```python
from build123d import *

# Parameters (mm, degrees)
SKETCH_2_R          = 6.05
SKETCH_2_R_2        = 1.6
EXTRUDE_1_DEPTH     = 3
SKETCH_2_3_R        = 1.6
EXTRUDE_2_DEPTH     = 8
SKETCH_3_R          = 1.65
EXTRUDE_4_DEPTH     = 3
SKETCH_5_R          = 3
CUT_EXTRUDE_1_DEPTH = 3.5
SKETCH_6_W          = 55.305281636
SKETCH_6_H          = 51.082077229
CUT_EXTRUDE_2_DEPTH = 82.174934555
FILLET_10_R         = 6
FILLET_11_R         = 5


with BuildPart() as part:
    # ｽｹｯﾁ2 → ﾎﾞｽ - 押し出し1 (new body)
    with BuildSketch(Plane.XY):
        with BuildLine():
            Line((-22.3, 23.9), (22.3, 23.9))
            Line((22.3, 23.9), (22.3, 38.9))
            Line((22.3, 38.9), (19.3, 38.9))
            ThreePointArc((19.3, 38.9), (0, 48.9), (-19.3, 38.9))
            Line((-19.3, 38.9), (-22.3, 38.9))
            Line((-22.3, 38.9), (-22.3, 23.9))
        make_face()
        with Locations((0, 36.4)):
            Circle(SKETCH_2_R, mode=Mode.SUBTRACT)
        with Locations((-9, 36.4)):
            Circle(SKETCH_2_R_2, mode=Mode.SUBTRACT)
        with Locations((9, 36.4)):
            Circle(SKETCH_2_R_2, mode=Mode.SUBTRACT)
    extrude(amount=-EXTRUDE_1_DEPTH)

    # ｽｹｯﾁ2<3> → ﾎﾞｽ - 押し出し2 (add)
    with BuildSketch(Plane.XY):
        with BuildLine():
            Line((22.3, 23.9), (-22.3, 23.9))
            Line((-22.3, 23.9), (-22.3, 14.9))
            Line((-22.3, 14.9), (-6.1, 14.9))
            ThreePointArc((-6.1, 14.9), (0, 21), (6.1, 14.9))
            Line((6.1, 14.9), (22.3, 14.9))
            Line((22.3, 14.9), (22.3, 23.9))
        make_face()
        with Locations((-17, 18.8)):
            Circle(SKETCH_2_3_R, mode=Mode.SUBTRACT)
        with Locations((17, 18.8)):
            Circle(SKETCH_2_3_R, mode=Mode.SUBTRACT)
    extrude(amount=-EXTRUDE_2_DEPTH)

    # ｽｹｯﾁ3 → ﾎﾞｽ - 押し出し4 (add)
    with BuildSketch(Plane.ZY.offset(22.3)):
        with BuildLine():
            Line((-8, 23.9), (-10.9, 23.9))
            Line((-10.9, 23.9), (-10.9, 16.120888862))
            Line((-10.9, 16.120888862), (-43, 16.120888862))
            ThreePointArc((-43, 16.120888862), (-46.752084661, 18.734576957), (-45.600779817, 23.159958513))
            ThreePointArc((-45.600779817, 23.159958513), (-25.707792424, 34.839146133), (-3, 38.9))
            Line((-3, 38.9), (-3, 23.9))
            Line((-3, 23.9), (-8, 23.9))
        make_face()
        with Locations(Location((-43, 20.120888862, 0), (0, 0, 270))):
            Circle(SKETCH_3_R, mode=Mode.SUBTRACT)
    extrude_4 = extrude(amount=-EXTRUDE_4_DEPTH)

    # ﾐﾗｰ11: ﾎﾞｽ - 押し出し4 across plane
    add(extrude_4.mirror(Plane(origin=(0, 0, 0), x_dir=(0, 0, 1), z_dir=(1, 0, 0))))

    # ｽｹｯﾁ5 → ｶｯﾄ - 押し出し1 (cut)
    with BuildSketch(Plane.XY):
        with Locations((-17, 18.8)):
            Circle(SKETCH_5_R)
        with Locations((17, 18.8)):
            Circle(SKETCH_5_R)
    extrude(amount=-CUT_EXTRUDE_1_DEPTH, mode=Mode.SUBTRACT)

    # ｽｹｯﾁ6 → ｶｯﾄ - 押し出し2 (cut, through all)
    with BuildSketch(Plane.ZY.offset(22.3)):
        with Locations((-38.552640818, 41.661927477)):
            Rectangle(SKETCH_6_W, SKETCH_6_H)
    extrude(amount=-CUT_EXTRUDE_2_DEPTH, mode=Mode.SUBTRACT)

    # ﾌｨﾚｯﾄ10
    # the kernel refuses this fillet: 6 mm, written as the material it adds along each edge
    with BuildSketch(Plane(origin=(19.3, 38.9, 0), x_dir=(-0.6205037663908469, 0.7842034658778125, 0), z_dir=(0, 0, -1))) as fillet_10_piece_1:
        with BuildLine():
            CenterArc((2.9106521, 5.991029767), FILLET_10_R, 218.352931503, 48.513653053)
            Line((-1.794568695, 2.268007169), (0, 0))
            ThreePointArc((0, 0), (1.29134257, 0.035319543), (2.582685141, 0))
        make_face()
    extrude(amount=3)
    with BuildSketch(Plane(origin=(-19.3, 38.9, 0), x_dir=(-1, 0, 0), z_dir=(0, 0, -1))) as fillet_10_piece_2:
        with BuildLine():
            CenterArc((2.892115717, 6), FILLET_10_R, 221.486346947, 48.513653053)
            ThreePointArc((-1.602565857, 2.025350639), (-0.77358522, 1.034591229), (0, 0))
            Line((0, 0), (2.892115717, 0))
        make_face()
    extrude(amount=3)

    # ﾌｨﾚｯﾄ11
    fillet_11_edges = [part.edges().sort_by_distance(p)[0] for p in [
        (19.3, 31.4, -3),
        (-19.3, 31.4, -3),
    ]]
    fillet(fillet_11_edges, radius=FILLET_11_R)


solid = part.part
```
Here's how the part is built. I have some questions about the finished solid (model axes, mm). A direction names the side the tool comes from. Give positions to 0.01 mm unless a question says otherwise; leave off trailing zeros. Write each loop counter-clockwise with the first axis right and the second up, starting at its lowest first coordinate (ties: lowest second). Pieces come first, ordered by that corner, then holes.
(1) Imagine slicing it at D-D, the plane z = -9.25. Write out the boundary of the cut face in (x, y), and give its area (3 significant figures).
Output values:
outline: (-22.3, 23.9) - (-19.3, 23.9) - (-19.3, 38.6) - (-22.3, 38.6) - close; (19.3, 23.9) - (22.3, 23.9) - (22.3, 38.6) - (19.3, 38.6) - close
area: 88.2 mm2
(2) Imagine slicing it at A-A, the plane y = 18.8. Write out the boundary of the cut face in (x, z), and give its area (3 significant figures).
Output values:
outline: (-22.3, -8) - (-18.6, -8) - (-18.6, -3.5) - (-20, -3.5) - (-20, 0) - (-22.3, 0) - close; (-15.4, -8) - (-4.69, -8) - (-4.69, 0) - (-14, 0) - (-14, -3.5) - (-15.4, -3.5) - close; (4.69, -8) - (15.4, -8) - (15.4, -3.5) - (14, -3.5) - (14, 0) - (4.69, 0) - close; (18.6, -8) - (22.3, -8) - (22.3, 0) - (20, 0) - (20, -3.5) - (18.6, -3.5) - close
area: 211 mm2
(3) Imagine slicing it at B-B, the plane z = -1. Write out the boundary of the cut face in (x, y).
Output values:
outline: (-22.3, 14.9) - (-6.1, 14.9) arc R6.1 cw to (6.1, 14.9) - (22.3, 14.9) - (22.3, 38.9) - (22.19, 38.9) arc R6 cw to (17.7, 40.93) arc R23.62 ccw to (-17.7, 40.93) arc R6 cw to (-22.19, 38.9) - (-22.3, 38.9) - close; hole circle Ø6 at (-17, 18.8); hole circle Ø3.2 at (-9, 36.4); hole circle Ø12.1 at (0, 36.4); hole circle Ø3.2 at (9, 36.4); hole circle Ø6 at (17, 18.8)
(4) If I drill on L1, parallel to Y at x = 0, z = -1.8; L2, parallel to X at y = 35, z = -9.75; L3, parallel to Z at x = 8, y = 20, over which ranges is the centre line in solid material (lowest first)?
Output values:
L1: y = 21 to 30.35, 42.45 to 48.9
L2: x = -22.3 to -19.3, 19.3 to 22.3
L3: z = -8 to 0
(5) Imagine slicing it at C-C, the plane x = 9. Write out the boundary of the cut face in (y, z).
Output values:
outline: (14.9, -8) - (23.9, -8) - (23.9, -3) - (34.8, -3) - (34.8, 0) - (14.9, 0) - close; (38, -3) - (47.12, -3) - (47.12, 0) - (38, 0) - close
(6) On a 3-axis mill with a long thin cutter (end or side, diameter ignored), from which of +Z, -Z, +X, -X, +Y, -Y can I reach the whole of each face in a straight line? I mean faces 1 (the face through (19.3, 31, -9)), 2 (the face through (-15.7, 17.5, -3.5)), 3 (the face through (-0.3, 21.5, -8)). Say none if no direction works.
Output values:
face 1: -Z, +Y, -Y
face 2: +Z
face 3: -Z, +X, -X, -Y
(7) Will these pins go through, and if not, where does the flat tip stop? pin 1 (3 mm diameter, centred on x = 15.5, y = 19.5, fed in from +Z); pin 2 (3.5 mm diameter, centred on x = -17, y = 18.8, fed in from -Z); pin 3 (3 mm diameter, centred on x = -16, y = 18, fed in from +Z); pin 4 (6 mm diameter, centred on x = -0.5, z = -7, fed in from +Y).
Output values:
pin 1: stops at z = 0
pin 2: stops at z = -8
pin 3: stops at z = -3.5
pin 4: stops at y = 23.9
(8) Thinking about a two-plate mould opening in X: for faces 4 (the face through (22.3, 27, -5)), 5 (the face through (0, 23.9, -5)), 6 (the face through (0.3, 48.9, -1.5)), which applies, pulls with the +X half, pulls with the -X half, needs draft (parallel to the pull), parting line crosses it, or undercut?
Output values:
face 4: pulls with the +X half
face 5: undercut
face 6: parting line crosses it
